```python
from build123d import *

# Parameters (mm, degrees)
CROQUIS2_W              = 53
CROQUIS2_H              = 98.6
SALIENTE_EXTRUIR1_DEPTH = 1.6
CROQUIS3_W              = 17.252718504
CROQUIS3_H              = 50.95570349
CROQUIS3_W_2            = 13.240458387
CROQUIS3_H_2            = 14.042910411
CROQUIS3_W_3            = 4.012260117
CROQUIS3_H_3            = 28.888272845
CROQUIS3_H_4            = 4.012260117
CROQUIS3_H_5            = 4.413486129
CROQUIS3_W_4            = 3.809203095
CROQUIS3_H_6            = 7.067484179
CROQUIS3_H_7            = 11.981054517
CROQUIS3_W_5            = 13.641684399
CROQUIS3_H_8            = 3.209808094
SALIENTE_EXTRUIR2_DEPTH = 8


with BuildPart() as part:
    # Croquis2 → Saliente-Extruir1 (new body)
    with BuildSketch(Plane(origin=(0, 0, 0), x_dir=(1, 0, 0), z_dir=(0, 1, 0))):
        Rectangle(CROQUIS2_W, CROQUIS2_H)
    extrude(amount=SALIENTE_EXTRUIR1_DEPTH)

    # Croquis3 → Saliente-Extruir2 (add)
    with BuildSketch(Plane(origin=(0, 1.6, 0), x_dir=(1, 0, 0), z_dir=(0, 1, 0))):
        with Locations((7.623294223, 5.81777717)):
            Rectangle(CROQUIS3_W, CROQUIS3_H)
        with Locations((-13.039845382, -34.706050015)):
            Rectangle(CROQUIS3_W_2, CROQUIS3_H_2)
        with Locations((-19.660074575, -3.410421099)):
            Rectangle(CROQUIS3_W_3, CROQUIS3_H_3)
        with Locations((7.623294223, 45.338539326)):
            Rectangle(CROQUIS3_W, CROQUIS3_H_4)
        with Locations((7.623294223, 37.113406084)):
            Rectangle(CROQUIS3_W, CROQUIS3_H_5)
        with Locations((21.567120139, 18.533688555)):
            Rectangle(CROQUIS3_W_4, CROQUIS3_H_6)
        with Locations((21.567120139, -3.4104211)):
            Rectangle(CROQUIS3_W_4, CROQUIS3_H_7)
        with Locations((7.623294223, -31.696854927)):
            Rectangle(CROQUIS3_W_5, CROQUIS3_H_8)
    extrude(amount=SALIENTE_EXTRUIR2_DEPTH)


solid = part.part
```
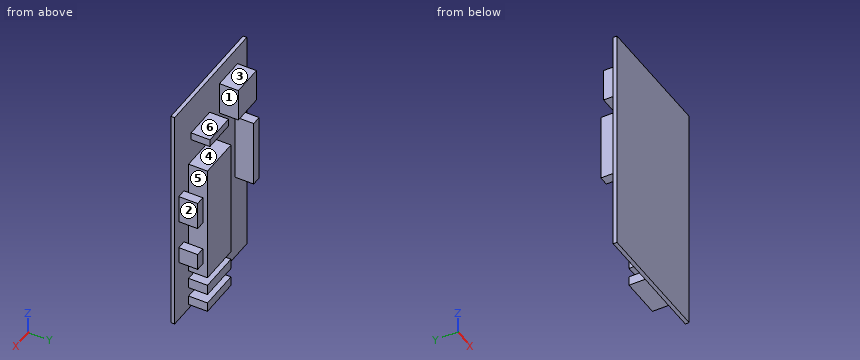
Work out the finished part from the listing and answer in its coordinate system (mm). Face numbers are marked on the shaded views. A direction names the side the tool comes from. Give positions to 0.01 mm unless a question says otherwise; leave off trailing zeros. Loops run counter-clockwise (first coordinate to the right, second up) from the corner with the lowest first, then second, coordinate; pieces in that order, holes last. Notation, with made-up numbers: M 51,-5.5 L 89,-5.5 A21 ccw 89,16.5 Z; hole C -9,-40 d3. An arc over 180 degrees is marked long. One line per item, written item: value. Start each with the question number.
1. Find the intervals of material crossed by probe 1 along Z at (x, y) = (1.5, 4); probe 2 along X at (y, z) = (5.5, 9); probe 3 along Z at (x, y) = (20, 3.75), in increasing order.
2. Each of these flat-tipped pins is pushed along its axis until it touches: P1, Ø3.5, axis at y = 3.5, z = -18.5, coming from the +X side; P2, Ø2, axis at y = 4, z = 2.5, coming from the -X side; P3, Ø4, axis at x = 5, y = 4, coming from the +Z side. Where does it stop, or does it pass through?
3. Find section B-B (x = 4.5). Give the vertices of the cut face in (y, z), and give its area (3 significant figures).
4. Which of the six approach directions +Z, -Z, +X, -X, +Y, -Y give full straight-line access (tool end or side, diameter ignored) to the marked faces 1, 2 and 3?
5. Find section A-A (y = 8.5). State how many separate pieces and enclosed holes the cut face has, and give its area (3 significant figures).
6. Find section D-D (x = -7.5). Give the vertices of the cut face in (y, z).
7. Determine the mould class of the marked faces 4, 5 and 6 for opening direction Z: released by +Z, released by -Z, zero draft, split by the parting line, or undercut.
8. Find section C-C (z = -25.5). Give the vertices of the cut face in (x, y).
Reported:
1. probe 1: z = -47.34 to -43.33, -39.32 to -34.91, -31.3 to 19.66, 30.09 to 33.3
1. probe 2: x = -21.67 to -17.65, -1 to 16.25, 19.66 to 23.47
1. probe 3: z = -22.07 to -15, -2.58 to 9.4
2. P1: stops at x = 23.47
2. P2: stops at x = -21.67
2. P3: stops at z = 33.3
3. outline: M 0,-49.3 L 1.6,-49.3 L 1.6,-47.34 L 9.6,-47.34 L 9.6,-43.33 L 1.6,-43.33 L 1.6,-39.32 L 9.6,-39.32 L 9.6,-34.91 L 1.6,-34.91 L 1.6,-31.3 L 9.6,-31.3 L 9.6,19.66 L 1.6,19.66 L 1.6,30.09 L 9.6,30.09 L 9.6,33.3 L 1.6,33.3 L 1.6,49.3 L 0,49.3 Z
3. area: 658 mm²
4. face 1: +Z, -Z, +Y
4. face 2: +Z, -Z, +X, +Y
4. face 3: +Z, +X, -X, +Y
5. separate pieces: 8
5. enclosed holes: 0
5. area: 1,440 mm²
6. outline: M 0,-49.3 L 1.6,-49.3 L 1.6,27.68 L 9.6,27.68 L 9.6,41.73 L 1.6,41.73 L 1.6,49.3 L 0,49.3 Z
7. face 4: undercut
7. face 5: zero draft
7. face 6: released by +Z
8. outline: M -26.5,0 L 26.5,0 L 26.5,1.6 L 16.25,1.6 L 16.25,9.6 L -1,9.6 L -1,1.6 L -26.5,1.6 Z
